Source: CAD feature listing. Evaluate the final solid. Frame: model axes, mm. Face numbers are marked on the shaded views. A direction names the side the tool comes from. Give positions to 0.01 mm unless a question says otherwise; leave off trailing zeros. Loops run counter-clockwise (first coordinate to the right, second up) from the corner with the lowest first, then second, coordinate; pieces in that order, holes last. Notation, with made-up numbers: (-34.75, 73) - (21.25, 73) arc R27 ccw to (21.25, 90) - close; hole circle Ø8 at (10.5, 86). An arc over 180 degrees is marked (long way). Put each result on its own line as item: value.
```python
from build123d import *

# Parameters (mm, degrees)
SKETCH_1_W               = 95
SKETCH_1_H               = 30.3
EXTRUDE_1_DEPTH          = 3.5
SKETCH_2_W               = 80.45
SKETCH_2_H               = 30.3
EXTRUDE_2_DEPTH          = 16.05
FILLET_1_R               = 5
CUT_EXTRUDE_1_DEPTH      = 54.553477945
CUT_EXTRUDE_1_DEPTH_BACK = 54.553477945
CUT_EXTRUDE_2_DEPTH      = 53.377237422
CUT_EXTRUDE_2_DEPTH_BACK = 53.377237422
SKETCH_4_R               = 1.75
SKETCH_5_R               = 1.725
EXTRUDE_3_DEPTH          = 9.45
MIRROR_2_COPY_1_SKETCH_R = 1.725
MIRROR_2_COPY_1_DEPTH    = 9.45


with BuildPart() as part:
    # Эскиз1 → Бобышка-Вытянуть1 (new body)
    with BuildSketch(Plane(origin=(0, 0, 0), x_dir=(1, 0, 0), z_dir=(0, 1, 0))):
        Rectangle(SKETCH_1_W, SKETCH_1_H)
    extrude(amount=EXTRUDE_1_DEPTH)

    # Эскиз2 → Бобышка-Вытянуть2 (add)
    with BuildSketch(Plane(origin=(0, 3.5, 0), x_dir=(1, 0, 0), z_dir=(0, 1, 0))):
        Rectangle(SKETCH_2_W, SKETCH_2_H)
    extrude(amount=EXTRUDE_2_DEPTH)

    # Скругление1
    fillet_1_edges = [part.edges().sort_by_distance(p)[0] for p in [
        (40.225, 11.525, 15.15),
        (40.225, 11.525, -15.15),
        (-40.225, 11.525, -15.15),
        (-40.225, 11.525, 15.15),
        (47.5, 1.75, 15.15),
        (-47.5, 1.75, 15.15),
        (-47.5, 1.75, -15.15),
        (47.5, 1.75, -15.15),
    ]]
    fillet(fillet_1_edges, radius=FILLET_1_R)

    # Эскиз3 → Вырез-Вытянуть1 (cut, two sides: drawn at the far end of the back side and taken through both)
    with BuildSketch(Plane(origin=(0, 19.55, 0), x_dir=(1, 0, 0), z_dir=(0, 1, 0)).offset(-CUT_EXTRUDE_1_DEPTH_BACK)):
        with BuildLine():
            Line((-32.775, 12.7), (32.775, 12.7))
            ThreePointArc((32.775, 12.7), (36.310533906, 11.235533906), (37.775, 7.7))
            Line((37.775, 7.7), (37.775, -7.7))
            ThreePointArc((37.775, -7.7), (36.310533906, -11.235533906), (32.775, -12.7))
            Line((32.775, -12.7), (-32.775, -12.7))
            ThreePointArc((-32.775, -12.7), (-36.310533906, -11.235533906), (-37.775, -7.7))
            Line((-37.775, -7.7), (-37.775, 7.7))
            ThreePointArc((-37.775, 7.7), (-36.310533906, 11.235533906), (-32.775, 12.7))
        make_face()
    extrude(amount=CUT_EXTRUDE_1_DEPTH + CUT_EXTRUDE_1_DEPTH_BACK, mode=Mode.SUBTRACT)

    # Эскиз4 → Вырез-Вытянуть2 (cut, two sides: drawn at the far end of the back side and taken through both)
    with BuildSketch(Plane(origin=(0, 3.5, 0), x_dir=(1, 0, 0), z_dir=(0, 1, 0)).offset(-CUT_EXTRUDE_2_DEPTH_BACK)):
        with Locations(Location((-43, 9, 0), (0, 0, 270))):
            Circle(SKETCH_4_R)
        with Locations(Location((43, 9, 0), (0, 0, 270))):
            Circle(SKETCH_4_R)
        with Locations(Location((-43, -9, 0), (0, 0, 270))):
            Circle(SKETCH_4_R)
        with Locations(Location((43, -9, 0), (0, 0, 270))):
            Circle(SKETCH_4_R)
    extrude(amount=CUT_EXTRUDE_2_DEPTH + CUT_EXTRUDE_2_DEPTH_BACK, mode=Mode.SUBTRACT)

    # Эскиз5 → Бобышка-Вытянуть3 (add)
    with BuildSketch(Plane.XZ):
        with BuildLine():
            Line((-37.775, 7.7), (-37.775, 4.2))
            Line((-37.775, 4.2), (-34.275, 4.2))
            ThreePointArc((-34.275, 4.2), (-30.739466094, 5.664466094), (-29.275, 9.2))
            Line((-29.275, 9.2), (-29.275, 12.7))
            Line((-29.275, 12.7), (-32.775, 12.7))
            ThreePointArc((-32.775, 12.7), (-36.310533906, 11.235533906), (-37.775, 7.7))
        make_face()
        with Locations(Location((-32.641070297, 7.616996928, 0), (0, 0, 270))):
            Circle(SKETCH_5_R, mode=Mode.SUBTRACT)
    extrude_3 = extrude(amount=-EXTRUDE_3_DEPTH)

    # Зеркальное отражение1: Бобышка-Вытянуть3 across plane
    add(extrude_3.mirror(Plane.XY))

    # Зеркальное отражение2: Бобышка-Вытянуть3 across plane
    add(extrude_3.mirror(Plane(origin=(0, 0, 0), x_dir=(0, 0, 1), z_dir=(1, 0, 0))))

    # Зеркальное отражение2 copy 1 sketch → Зеркальное отражение2 copy 1 (add)
    with BuildSketch(Plane(origin=(0, 0, 0), x_dir=(-1, 0, 0), z_dir=(0, -1, 0))):
        with BuildLine():
            Line((-37.775, 7.7), (-37.775, 4.2))
            Line((-37.775, 4.2), (-34.275, 4.2))
            ThreePointArc((-34.275, 4.2), (-30.739466094, 5.664466094), (-29.275, 9.2))
            Line((-29.275, 9.2), (-29.275, 12.7))
            Line((-29.275, 12.7), (-32.775, 12.7))
            ThreePointArc((-32.775, 12.7), (-36.310533906, 11.235533906), (-37.775, 7.7))
        make_face()
        with Locations(Location((-32.641070297, 7.616996928, 0), (0, 0, 270))):
            Circle(MIRROR_2_COPY_1_SKETCH_R, mode=Mode.SUBTRACT)
    extrude(amount=-MIRROR_2_COPY_1_DEPTH)


solid = part.part
```
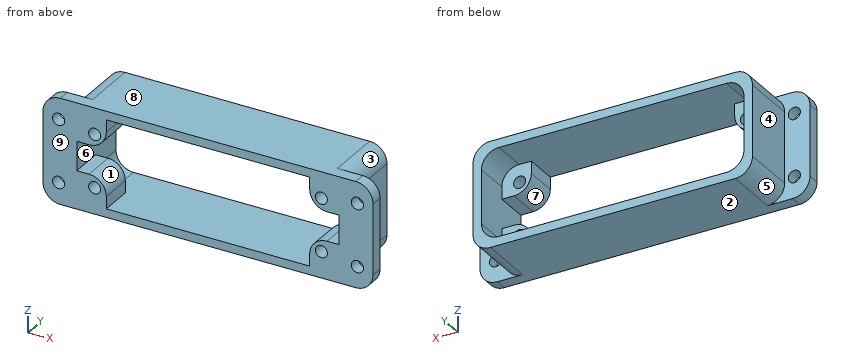
1) Section query A-A, the plane x = 21. Output: boundary loops of the cut face in (y, z).
Check result:
outline: (0, -15.15) - (19.55, -15.15) - (19.55, -12.7) - (0, -12.7) - close; (0, 12.7) - (19.55, 12.7) - (19.55, 15.15) - (0, 15.15) - close
2) Section query B-B, the plane y = 15.75. Output: boundary loops of the cut face in (x, z) (3 decimals), plus the area to 3 significant figures.
Check result:
outline: (-40.225, -10.15) arc R5 ccw to (-35.225, -15.15) - (35.225, -15.15) arc R5 ccw to (40.225, -10.15) - (40.225, 10.15) arc R5 ccw to (35.225, 15.15) - (-35.225, 15.15) arc R5 ccw to (-40.225, 10.15) - close; hole (-37.775, -7.7) arc R5 ccw to (-32.775, -12.7) - (32.775, -12.7) arc R5 ccw to (37.775, -7.7) - (37.775, 7.7) arc R5 ccw to (32.775, 12.7) - (-32.775, 12.7) arc R5 ccw to (-37.775, 7.7) - close
area: 519 mm²
3) Section query C-C, the plane y = 2.5. State how many separate pieces and enclosed holes the cut face has, plus the area to 3 significant figures.
Check result:
separate pieces: 1
enclosed holes: 9
area: 1,130 mm²
4) Mould query, pull axis X, two halves, no side actions, for the marked faces 1, 2, 3 and 4. Classes: pulls with the +X half, pulls with the -X half, needs draft (parallel to the pull), parting line crosses it, or undercut.
Check result:
face 1: undercut
face 2: needs draft
face 3: pulls with the +X half
face 4: pulls with the -X half
5) Material intervals for line 1 along X through (y, z) = (15.75, 7.5) (3 decimals); line 2 along Z through (x, y) = (32.5, 1.75); line 3 along X through (y, z) = (1.05, -9), sorted ascending. Write a range as [from, to].
Check result:
line 1: [-40.225, -37.775], [37.775, 40.225]
line 2: [-15.15, -9.34], [-5.9, -4.53], [4.53, 5.9], [9.34, 15.15]
line 3: [-47.5, -44.75], [-41.25, -33.67], [-31.61, -29.28], [29.28, 31.61], [33.67, 41.25], [44.75, 47.5]
6) Access query for the marked faces 5, 6, 7, 8 and 9. Directions: +Z, -Z, +X, -X, +Y, -Y. A direction counts if a zero-diameter tool reaches every point of the face in a straight line with its end or side. Return the directions, or none.
Check result:
face 5: -Z, -X, +Y
face 6: +Y
face 7: +Y, -Y
face 8: +Z, +X, -X, +Y, -Y
face 9: +Z, -Z, +X, -X, -Y
7) Pin query (flat end, axial travel): P1, Ø5, axis at y = 17.5, z = 6.5, coming from the +X side (3 decimals); P2, Ø4, axis at y = 14, z = 1.5, coming from the -X side (3 decimals); P3, Ø3, axis at x = 43, z = -9, coming from the +Y side; P4, Ø1, axis at x = -33.5, z = 9, coming from the +Y side. Return the tip coordinate at first contact, or that it passes through.
Check result:
P1: x = 40.225
P2: x = -40.225
P3: through
P4: y = 9.45
